from build123d import *

# Parameters (mm, degrees)
SKETCH2_R          = 66.009585634
CUT_EXTRUDE1_DEPTH = 23
SKETCH4_R          = 31.856181498
CUT_EXTRUDE2_DEPTH = 17.7
SKETCH5_R          = 32.987885215
CUT_EXTRUDE3_DEPTH = 17.7


with BuildPart() as part:
    # Sketch1 → Revolve1 (revolve)
    with BuildSketch(Plane.XY):
        Polygon((0, -24.15), (12.7, -24.15), (12.7, -20.6), (62.8, -20.6), (78, -20.6), (78, -23.722326479), (58.4, -24.15), (58.4, -28.6), (40.7, -28.6), (40.7, -38), (17.7, -38), (17.7, -28.6), (0, -28.6), align=None)
    revolve(axis=Axis((0, 0, 0), (1, 0, 0)))

    # Sketch2 → Cut-Extrude1 (cut)
    with BuildSketch(Plane(origin=(40.7, 0, 0), x_dir=(0, 0, -1), z_dir=(1, 0, 0))):
        Circle(SKETCH2_R)
        Polygon((0, 38.42492311), (-27.170523698, 27.170523698), (-38.42492311, 0), (-27.170523698, -27.170523698), (0, -38.42492311), (27.170523698, -27.170523698), (38.42492311, 0), (27.170523698, 27.170523698), align=None, mode=Mode.SUBTRACT)
    extrude(amount=-CUT_EXTRUDE1_DEPTH, mode=Mode.SUBTRACT)

    # Sketch4 → Cut-Extrude2 (cut)
    with BuildSketch(Plane.ZY):
        Circle(SKETCH4_R)
        Polygon((1.020288253, 28.665241383), (-19.547933824, 20.990839308), (-28.665241383, 1.020288253), (-20.990839308, -19.547933824), (-1.020288253, -28.665241383), (19.547933824, -20.990839308), (28.665241383, -1.020288253), (20.990839308, 19.547933824), align=None, mode=Mode.SUBTRACT)
    extrude(amount=-CUT_EXTRUDE2_DEPTH, mode=Mode.SUBTRACT)

    # Sketch5 → Cut-Extrude3 (cut)
    with BuildSketch(Plane(origin=(58.4, 0, 0), x_dir=(0, 0, -1), z_dir=(1, 0, 0))):
        Circle(SKETCH5_R)
        Polygon((0.892984101, 28.66948955), (-19.640955361, 20.903825587), (-28.66948955, 0.892984101), (-20.903825587, -19.640955361), (-0.892984101, -28.66948955), (19.640955361, -20.903825587), (28.66948955, -0.892984101), (20.903825587, 19.640955361), align=None, mode=Mode.SUBTRACT)
    extrude(amount=-CUT_EXTRUDE3_DEPTH, mode=Mode.SUBTRACT)


solid = part.part
The listing builds one solid part. Answer for the finished solid, in the listing's coordinates (mm). A direction names the side the tool comes from. Coordinates: 2 decimals unless noted, no trailing zeros. Loops run counter-clockwise (first coordinate to the right, second up) from the corner with the lowest first, then second, coordinate; pieces in that order, holes last.
1) Find the intervals of material crossed by L1, parallel to Z at x = 36.5, y = 0; L2, parallel to X at y = -19.5, z = -26, in increasing order.
2) Find section B-B on x = 16.5. Write down the section's boundary in (y, z).
3) A tool of negligible diameter and unlimited length cuts with its end or side. For faces 5 (the face through (8.73, 24.88, -9.12)), 6 (the face through (49.67, 24.84, 9.23)), 7 (the face through (49.67, -24.09, 11.04)), 8 (the face through (49.67, 24.09, -11.04)), from which of +Z, -Z, +X, -X, +Y, -Y can it reach the whole face along a straight path? Write none if from no direction.
4) Find section A-A on x = 34. Write down the section's boundary in (y, z).
5) Find section D-D on x = 66. Write down the section's boundary in (y, z), then the cut area to 3 significant figures.
6) Flat-ended cylindrical pins translate along their axes: pin 1 Ø10 at (x, z) = (51.5, -6.5) entering from -Y; pin 2 Ø6 at (x, z) = (18, -29.5) entering from -Y; pin 3 Ø4 at (x, z) = (23.5, 19) entering from +Y; pin 4 Ø24.5 at (y, z) = (0, 0) entering from -X. Find the tip coordinate at first contact, or state that the pin passes through.
7) Determine the mould class of faces 1 (the face through (8.726, -24.044, -11.143)), 2 (the face through (29.36, -13.41, 32.87)), 3 (the face through (68.06, 5.19, 23.37)), 4 (the face through (6.439, 24.127, -1.062)) for opening direction Z: pulls with the +Z half, pulls with the -Z half, needs draft (parallel to the pull), parting line crosses it, or undercut.
8) Find section C-C on y = 31.5. Write down the section's boundary in (x, z).
Values:
1. L1: z = -38 to -20.6, 20.6 to 38
1. L2: x = 17.7 to 40.7
2. outline: (-28.59, -0.81) arc R28.6 ccw to (-28.57, -1.22) - (-19.64, -20.79) arc R28.6 ccw to (-19.34, -21.07) - (0.81, -28.59) arc R28.6 ccw to (1.22, -28.57) - (20.79, -19.64) arc R28.6 ccw to (21.07, -19.34) - (28.59, 0.81) arc R28.6 ccw to (28.57, 1.22) - (19.64, 20.79) arc R28.6 ccw to (19.34, 21.07) - (-0.81, 28.59) arc R28.6 ccw to (-1.22, 28.57) - (-20.79, 19.64) arc R28.6 ccw to (-21.07, 19.34) - close; hole circle Ø41.2 at (0, 0)
3. face 5: -Z, -X, +Y
3. face 6: +Z, +X, +Y
3. face 7: +Z, +X, -Y
3. face 8: -Z, +X, +Y
4. outline: (-37.99, -1.06) - (-27.61, -26.11) arc R38 ccw to (-26.11, -27.61) - (-1.06, -37.99) arc R38 ccw to (1.06, -37.99) - (26.11, -27.61) arc R38 ccw to (27.61, -26.11) - (37.99, -1.06) arc R38 ccw to (37.99, 1.06) - (27.61, 26.11) arc R38 ccw to (26.11, 27.61) - (1.06, 37.99) arc R38 ccw to (-1.06, 37.99) - (-26.11, 27.61) arc R38 ccw to (-27.61, 26.11) - (-37.99, 1.06) arc R38 ccw to start; hole circle Ø41.2 at (0, 0)
5. outline: circle Ø47.97 at (0, 0); hole circle Ø41.2 at (0, 0)
5. area: 474 mm2
6. pin 1: stops at y = -27.76
6. pin 2: stops at y = -27.24
6. pin 3: stops at y = 31.38
6. pin 4: passes through
7. face 1: pulls with the -Z half
7. face 2: pulls with the +Z half
7. face 3: parting line crosses it
7. face 4: undercut
8. outline: (17.7, -16.72) - (40.7, -16.72) - (40.7, 16.72) - (17.7, 16.72) - close
